The listing builds one solid part. Answer for the finished solid, in the listing's coordinates (mm). Face numbers are marked on the shaded views. A direction names the side the tool comes from. Coordinates: 2 decimals unless noted, no trailing zeros. Order: outer loops, then holes, each group sorted by start corner. A loop starts at its lowest first (then second) coordinate and runs counter-clockwise, first axis right, second up.
from build123d import *

# Parameters (mm, degrees)
F0_W      = 63.5
F0_H      = 15
F1_DEPTH  = 1.5
F2_W      = 10
F2_H      = 8
F3_DEPTH  = 1.5
F4_W      = 12
F4_H      = 7.5
F5_DEPTH  = 1.501
F6_R      = 1.5
F7_DEPTH  = 1.501
F8_W      = 10.7
F8_H      = 0.5
F9_DEPTH  = 15.001
F10_W     = 2
F10_H     = 1.5
F11_DEPTH = 23.001
F12_W     = 8
F12_H     = 23
F13_DEPTH = 1
F14_R     = 2
F15_R     = 0.5


with BuildPart() as f1:
    # F0 (on Front) → F1 (new body)
    with BuildSketch(Plane.XZ):
        with Locations((-6.75, 0)):
            Rectangle(F0_W, F0_H)
    extrude(amount=F1_DEPTH)

    # F2 (on face) → F3 (join, through all)
    with BuildSketch(Plane.XZ.offset(1.5)):
        with Locations((20, -11.5)):
            Rectangle(F2_W, F2_H)
    extrude(amount=-F3_DEPTH)

    # F4 (on face) → F5 (cut, through all)
    with BuildSketch(Plane.XZ.offset(1.5)):
        with Locations((-9.3, -3.75)):
            Rectangle(F4_W, F4_H)
    extrude(amount=-F5_DEPTH, mode=Mode.SUBTRACT)

    # F6 (on face) → F7 (cut, through all)
    with BuildSketch(Plane.XZ.offset(1.5)):
        with Locations((-34, 0)):
            Circle(F6_R)
    extrude(amount=-F7_DEPTH, mode=Mode.SUBTRACT)

    # F8 (on face) → F9 (cut, through all)
    with BuildSketch(Plane(origin=(0, 0, -7.5), x_dir=(1, 0, 0), z_dir=(0, 0, -1))):
        with Locations((-33.15, 1.25)):
            Rectangle(F8_W, F8_H)
    extrude(amount=-F9_DEPTH, mode=Mode.SUBTRACT)

    # F10 (on face) → F11 (cut, through all)
    with BuildSketch(Plane(origin=(0, 0, -15.5), x_dir=(1, 0, 0), z_dir=(0, 0, -1))):
        with Locations((24, 0.75)):
            Rectangle(F10_W, F10_H)
    extrude(amount=-F11_DEPTH, mode=Mode.SUBTRACT)

    # F12 (on face) → F13 (join)
    with BuildSketch(Plane(origin=(0, 0, 0), x_dir=(-1, 0, 0), z_dir=(0, 1, 0))):
        with Locations((-19, -4)):
            Rectangle(F12_W, F12_H)
    extrude(amount=F13_DEPTH)

    # F14
    f14_edges = [f1.edges().sort_by_distance(p)[0] for p in [
        (15, -0.25, -15.5),
        (23, -0.25, -15.5),
        (23, -0.25, 7.5),
        (-3.3, -0.75, -7.5),
        (-15.3, -0.75, -7.5),
    ]]
    fillet(f14_edges, radius=F14_R)

    # F15
    f15_edges = [f1.edges().sort_by_distance(p)[0] for p in [
        (23, 1, -4),
        (23, -1.5, -4),
    ]]
    fillet(f15_edges, radius=F15_R)


solid = f1.part
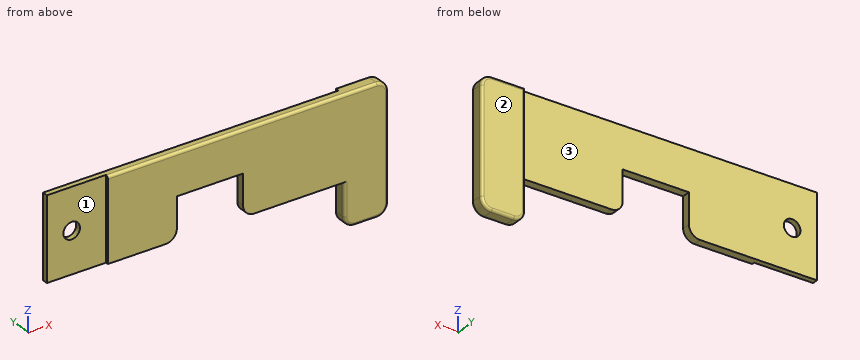
(1) Find section A-A on y = -0.5. Determine the outline of the cut face in (x, z), then the cut area to 3 significant figures.
(2) Find section B-B on z = -4. Determine the outline of the cut face in (x, y), then the cut area to 3 significant figures.
(3) A tool of negligible diameter and unlimited length cuts with its end or side. For the marked faces 1, 2 and 3, from which of +Z, -Z, +X, -X, +Y, -Y can it reach the whole face along a straight path? Write none if from no direction.
(4) Find section D-D on x = 5.5. Determine the outline of the cut face in (y, z), then the cut area to 3 significant figures.
(5) Find the intervals of material crossed by probe 1 along Z at (x, y) = (-34, -0.25); probe 2 along X at (y, z) = (-0.1, -2.5); probe 3 along X at (y, z) = (-0.6, -10), in increasing order.
(6) Given pin 1 Ø0.8 at (x, y) = (3.5, -1) entering from -Z; pin 2 Ø1 at (x, z) = (-31, -3) entering from +Y; pin 3 Ø3 at (x, z) = (-32, -3) entering from -Y, each flat-ended and moving along its own axis, determine where each tip first touches the part or whether it passes through.
(7) Find section C-C on x = -34. Determine the outline of the cut face in (y, z), then the cut area to 3 significant figures.
Resolved:
1. outline: (-38.5, -7.5) - (-17.3, -7.5) arc R2 ccw to (-15.3, -5.5) - (-15.3, 0) - (-3.3, 0) - (-3.3, -5.5) arc R2 ccw to (-1.3, -7.5) - (15, -7.5) - (15, -13.5) arc R2 ccw to (17, -15.5) - (21, -15.5) arc R2 ccw to (23, -13.5) - (23, 5.5) arc R2 ccw to (21, 7.5) - (-38.5, 7.5) - close; hole circle Ø3 at (-34, 0)
1. area: 885 mm2
2. outline: (-38.5, -1) - (-27.8, -1) - (-27.8, -1.5) - (-15.3, -1.5) - (-15.3, 0) - (-38.5, 0) - close; (-3.3, -1.5) - (22.5, -1.5) arc R0.5 ccw to (23, -1) - (23, 0.5) arc R0.5 ccw to (22.5, 1) - (15.5, 1) arc R0.5 ccw to (15, 0.5) - (15, 0) - (-3.3, 0) - close
2. area: 76.7 mm2
3. face 1: +Z, -Z, -X, -Y
3. face 2: +Z, -Z, +X, -X, +Y
3. face 3: +Z, -Z, -X, +Y
4. outline: (-1.5, -7.5) - (0, -7.5) - (0, 7.5) - (-1, 7.5) arc R0.5 ccw to (-1.5, 7) - close
4. area: 22.4 mm2
5. probe 1: z = -7.5 to -1.5, 1.5 to 7.5
5. probe 2: x = -38.5 to -15.3, -3.3 to 23
5. probe 3: x = 15 to 23
6. pin 1: stops at z = -7.5
6. pin 2: stops at y = 0
6. pin 3: stops at y = -1
7. outline: (-1, -7.5) - (0, -7.5) - (0, -1.5) - (-1, -1.5) - close; (-1, 1.5) - (0, 1.5) - (0, 7.5) - (-1, 7.5) - close
7. area: 12.0 mm2
